Autodesk Inventor part; units mm, degrees
ref_plane "YZ Plane" through (0, 0, 0) normal (1, 0, 0) x (0, 1, 0)
ref_plane "XZ Plane" through (0, 0, 0) normal (0, 1, 0) x (-1, 0, 0)
ref_plane "XY Plane" through (0, 0, 0) normal (0, 0, 1) x (1, 0, 0)
sketch "Szkic1" plane through (0, 0, 0) normal (1, 0, 0) x (0, 1, 0)
  circle A0 centre (0, 0) radius 7
  circle A1 centre (0, 0) radius 1.5
  line L0 (0, 1.5) -> (0, -1.0846)
  line L1 (-1, 1.9718) -> (-1, -1.0846)
  line L2 (8, 0) -> (-8, 0)
  line L3 (-8, 0) -> (-8, -1)
  line L4 (-8, -1) -> (8, -1)
  line L5 (8, -1) -> (8, 0)
  line L6 (8, 0) -> (-8, 0)
  line L7 (-8, 0) -> (-8, 1)
  line L8 (-8, 1) -> (8, 1)
  line L9 (8, 1) -> (8, 0)
  line L10 (0, 8) -> (1, 8)
  line L11 (1, 8) -> (1, -8)
  line L12 (1, -8) -> (0, -8)
  line L13 (0, 8) -> (-1, 8)
  line L14 (-1, 8) -> (-1, -8)
  line L15 (-1, -8) -> (0, -8)
  line L16 (0, -8) -> (0, 8)
  point P0 (-1, -1.118)
  point P1 (-1, 1.118)
  point P2 (-6.9282, -1)
  point P3 (-6.9282, 1)
  point P4 (1, -6.9282)
  point P5 (-1, -6.9282)
  point P6 (6.9282, 1)
  point P7 (6.9282, -1)
  point P8 (-1, 6.9282)
  point P9 (1, 6.9282)
  dimension "d1" = 3
  dimension "d0" = 14
  dimension "d2" = 1
  dimension "d14" = 16
  dimension "d16" = 16
  dimension "d18" = 2
  dimension "d19" = 2
sketch "Szkic2" plane through (0, 0, 0) normal (0, 0, 1) x (1, 0, 0)
  line L0 (0, 0) -> (5, 0)
  line L1 (5, 0) -> (5, 7)
  line L2 (5, 7) -> (0, 7)
  line L3 (0, 7) -> (0, 0)
  line L4 (0, 0) -> (-5, 0)
  line L5 (-5, 0) -> (-5, 7)
  line L6 (-5, 7) -> (0, 7)
  line L7 (0, 7) -> (0, 0)
  line L8 (0, 0) -> (5, 0)
  line L9 (5, 0) -> (5, -7)
  line L10 (5, -7) -> (0, -7)
  line L11 (0, -7) -> (0, 0)
  line L12 (0, 0) -> (-5, 0)
  line L13 (-5, 0) -> (-5, -7)
  line L14 (-5, -7) -> (0, -7)
  line L15 (0, -7) -> (0, 0)
  line L16 (5, 7) -> (4, 7)
  line L17 (4, 7) -> (4, 8)
  line L18 (4, 8) -> (5, 8)
  line L19 (5, 8) -> (5, 7)
  line L20 (3, 7) -> (2, 7)
  line L21 (2, 7) -> (2, 8)
  line L22 (2, 8) -> (3, 8)
  line L23 (3, 8) -> (3, 7)
  line L24 (-5, 7) -> (-4, 7)
  line L25 (-4, 7) -> (-4, 8)
  line L26 (-4, 8) -> (-5, 8)
  line L27 (-5, 8) -> (-5, 7)
  line L28 (-3, 7) -> (-2, 7)
  line L29 (-2, 7) -> (-2, 8)
  line L30 (-2, 8) -> (-3, 8)
  line L31 (-3, 8) -> (-3, 7)
  dimension "d3" = 5
  dimension "d4" = 7
  dimension "d5" = 10
  dimension "d6" = 14
  dimension "d7" = 1
  dimension "d8" = 1
  dimension "d9" = 1
  dimension "d10" = 1
  dimension "d11" = 1
  dimension "d12" = 1
  dimension "d13" = 1
extrude "Wyciągnięcie proste1" add sketch "Szkic1" along normal mid plane 10 contours L2 A1 L8 A0 | A0 L4 A1 L2 | L8 A1 L11 A0 | A0 L11 A1 L4 | L11 A1 L16 A0 | A0 L16 A1 L11 | L16 A1 L1 L14 A0 | A0 L14 A1 L16 | L14 L1 A1 L8 A0 | A0 L4 A1 L14 | L2 A1 L8 L1 | L1 L4 A1 L2 | L8 A1 L2 A0 | L1 L8 A1 | A0 L2 A1 L4 | A1 L4 L1 L14
extrude "Wyciągnięcie proste2" add sketch "Szkic1" along normal mid plane 4 contours L2 L5 L4 A0 | A0 L8 L9 L2 | A0 L16 L10 L11 | L11 L12 L16 A0 | A0 L14 L13 L16 | L16 L15 L14 A0 | A0 L2 L7 L8 | L4 L3 L2 A0
revolve "Obrót1" add sketch "Szkic2" angle 360 about axis through (0, 0, 0) along (1, 0, 0) contours L2 L17 L18 L19 | L21 L22 L23 L2 | L6 L31 L30 L29 | L27 L26 L25 L6
properties part number "lepszy kolo"
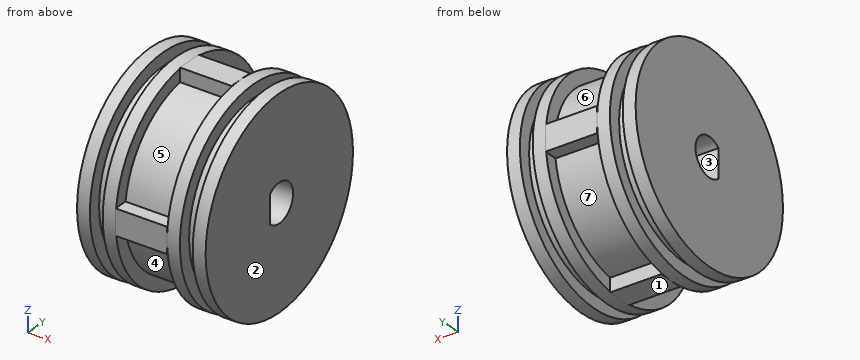
Work out the finished part from the listing and answer in its coordinate system (mm). Face numbers are marked on the shaded views. A direction names the side the tool comes from. Round coordinates to 2 decimals unless told otherwise and drop trailing zeros. Loops run counter-clockwise (first coordinate to the right, second up) from the corner with the lowest first, then second, coordinate; pieces in that order, holes last. Notation, with made-up numbers: M 16,89.5 L 43,89.5 A14 cw 43,108.5 Z; hole C 1.5,11.5 d6. An arc over 180 degrees is marked long. Use CSV: the item, a comma, the result in double quotes.
Q1. Section D-D, the plane z = 6 is taken. Determine the outline of the cut face in (x, y).
Determined:
outline,"M -5,-5.29 L -4,-5.29 L -4,-3.61 L -3,-3.61 L -3,-5.29 L -2,-5.29 L -2,-3.61 L 2,-3.61 L 2,-5.29 L 3,-5.29 L 3,-3.61 L 4,-3.61 L 4,-5.29 L 5,-5.29 L 5,5.29 L 4,5.29 L 4,3.61 L 3,3.61 L 3,5.29 L 2,5.29 L 2,3.61 L -2,3.61 L -2,5.29 L -3,5.29 L -3,3.61 L -4,3.61 L -4,5.29 L -5,5.29 Z"
Q2. Each of these flat-tipped pins is pushed along its axis until it touches: pin 1 (0.5 mm diameter, centred on x = 1, y = 7.5, fed in from -Z); pin 2 (1.5 mm diameter, centred on x = -0.5, z = -5, fed in from +Y); pin 3 (3.5 mm diameter, centred on y = 0, z = 0, fed in from -X); pin 4 (5 mm diameter, centred on x = 2, y = -4, fed in from +Z). Where does it stop, or does it pass through?
Determined:
pin 1,"z = -1"
pin 2,"y = 5.56"
pin 3,"x = -5"
pin 4,"z = 7.86"
Q3. Consider L1, parallel to X at y = -5.5, z = 5; L2, parallel to Y at x = 1.5, z = 0; L3, parallel to Z at x = 1, y = 0. Determine where each line is inside the solid, lowest interval first.
Determined:
L1,"-5 to -4, -3 to -2, 2 to 3, 4 to 5"
L2,"-8 to -1, 1.5 to 8"
L3,"-8 to -1.5, 1.5 to 8"
Q4. The mould has two halves that part along Z. Classify the marked faces 1, 2 and 3: pulls with the +Z half, pulls with the -Z half, needs draft (parallel to the pull), parting line crosses it, or undercut.
Determined:
face 1,"pulls with the -Z half"
face 2,"needs draft"
face 3,"undercut"
Q5. Section C-C, the plane y = 3.5 is taken. Determine the outline of the cut face in (x, z), then the cut area to 3 significant figures.
Determined:
outline,"M -5,-7.19 L -4,-7.19 L -4,-6.06 L -3,-6.06 L -3,-7.19 L -2,-7.19 L -2,-6.06 L 2,-6.06 L 2,-7.19 L 3,-7.19 L 3,-6.06 L 4,-6.06 L 4,-7.19 L 5,-7.19 L 5,7.19 L 4,7.19 L 4,6.06 L 3,6.06 L 3,7.19 L 2,7.19 L 2,6.06 L -2,6.06 L -2,7.19 L -3,7.19 L -3,6.06 L -4,6.06 L -4,7.19 L -5,7.19 Z"
area,"130 mm2"
Q6. Section B-B, the plane x = 0.5 is taken. Determine the outline of the cut face in (y, z), then the cut area to 3 significant figures.
Determined:
outline,"M -8,-1 L -6.93,-1 A7 ccw -1,-6.93 L -1,-8 L 1,-8 L 1,-6.93 A7 ccw 6.93,-1 L 8,-1 L 8,1 L 6.93,1 A7 ccw 1,6.93 L 1,8 L -1,8 L -1,6.93 A7 ccw -6.93,1 L -8,1 Z; hole M -1,-1.12 A1.5 ccw long -1,1.12 Z"
area,"156 mm2"
Q7. A tool of negligible diameter and unlimited length cuts with its end or side. For the marked faces 4, 5, 6 and 7, from which of +Z, -Z, +X, -X, +Y, -Y can it reach the whole face along a straight path? Write none if from no direction.
Determined:
face 4,"-Z, -Y"
face 5,"+Z, -Y"
face 6,"+Z, +Y"
face 7,"-Z, +Y"
